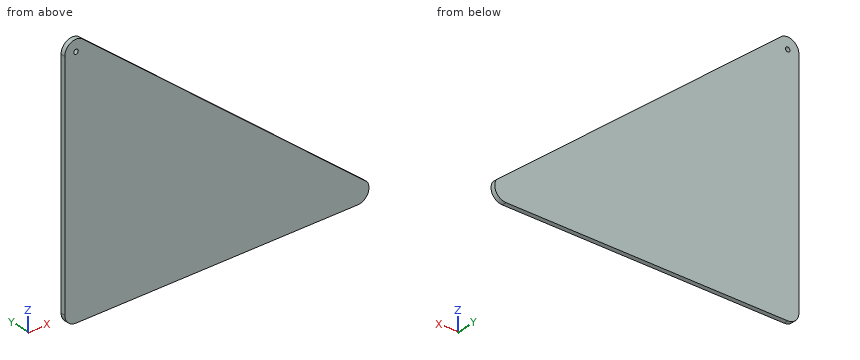
from build123d import *

# Parameters (mm, degrees)
ESQUISSE1_R        = 1
BOSS_EXTRU_2_DEPTH = 2


with BuildPart() as part:
    # Esquisse1 → Boss.-Extru.2 (new body)
    with BuildSketch(Plane(origin=(0, 0, 0), x_dir=(1, 0, 0), z_dir=(0, 1, 0))):
        with BuildLine():
            Line((129.333821146, 100.5), (2.5, -4.330127019))
            ThreePointArc((2.5, -4.330127019), (-2.5, -4.330127019), (-5, 0))
            Line((-5, 0), (-5, 103))
            ThreePointArc((-5, 103), (-3.535533906, 106.535533906), (0, 108))
            Line((0, 108), (125.003694127, 108))
            ThreePointArc((125.003694127, 108), (129.333821146, 105.5), (129.333821146, 100.5))
        make_face()
        Circle(ESQUISSE1_R, mode=Mode.SUBTRACT)
    extrude(amount=BOSS_EXTRU_2_DEPTH)


solid = part.part
The model under review builds one solid part; all positions refer to its coordinate system, in mm. Round coordinates to 2 decimals unless told otherwise and drop trailing zeros. Order: outer loops, then holes, each group sorted by start corner. A loop starts at its lowest first (then second) coordinate and runs counter-clockwise, first axis right, second up. Notation, with made-up numbers: (-26, 65.5) -> (-6, 65.5) arc R17 cw to (-6, 80.5) -> close; hole circle Ø5 at (-16, 15). An arc over 180 degrees is marked (long way). Use CSV: the item, a comma, the result in double quotes. Start each with the question number.
(1) Insertion check: pin 1 (10 mm diameter, centred on x = 21.5, z = -18, fed in from -Y); pin 2 (1 mm diameter, centred on x = 55, y = 1, fed in from +Z). Each pin has a flat end and moves straight along its axis. Give the tip position at first contact, or say it passes through.
(2) Consider section C-C on x = 49. Write out the cut boundary in (y, z), and give its area (3 significant figures).
(3) Consider section B-B on z = -61.5. Write out the cut boundary in (x, y).
(4) Consider section A-A on y = 1.25. Write out the cut boundary in (x, z).
(5) Wall thickness on probe 1 along X at (y, z) = (0.45, 0); probe 2 along Z at (x, y) = (120.5, 0.45); probe 3 along Z at (x, y) = (75, 1.7): over which ranges is each line inside the solid? List them lowest first. Write a range as from..to.
Responses:
1,pin 1,"y = 0"
1,pin 2,"z = -38.65"
2,outline,"(0, -108) -> (2, -108) -> (2, -34.1) -> (0, -34.1) -> close"
2,area,"148 mm²"
3,outline,"(-5, 0) -> (82.15, 0) -> (82.15, 2) -> (-5, 2) -> close"
4,outline,"(-5, -103) arc R5 ccw to (0, -108) -> (125, -108) arc R5 ccw to (129.33, -100.5) -> (2.5, 4.33) arc R5 ccw to (-5, 0) -> close; hole circle Ø2 at (0, 0)"
5,probe 1,"-5..-1, 1..7.74"
5,probe 2,"-108..-93.2"
5,probe 3,"-108..-55.59"
